Job drawing, mm, ordinate dimensions from the low corner. One solid piece. A direction names the side the tool comes from. Round coordinates to 2 decimals unless told otherwise and drop trailing zeros. Loops run counter-clockwise (first coordinate to the right, second up) from the corner with the lowest first, then second, coordinate; pieces in that order, holes last.
1) Drop a flat-ended pin along its axis: P1, Ø8, axis at x = 47.5, y = 28, coming from the +Z side. Give the stop position or say it passes through.
2) Band-saw the part on C-C, the plane y = 28. Write the cut outline in (x, z).
3) Band-saw the part on D-D, the plane x = 66. Write the cut outline in (y, z) (3 decimals).
4) 3-axis set-ups, long thin cutter, end or side, ignore diameter. For the marked faces 1 and 2: which of +Z, -Z, +X, -X, +Y, -Y reach the whole face in a straight line?
5) Mould opens along X. For the marked faces 3, 4, 5 and 6 say: +X half, -X half, draft (parallel to the pull), parting line (faces both ways), or undercut.
6) Probe line 1 (Y direction, x = 66, z = 2.95); line 2 (Y direction, x = 13, z = 1.65); line 3 (Y direction, x = 38, z = 4.5). List the from-to ranges inside material, lowest first.
7) Band-saw the part on B-B, the plane z = 3.4. Write the cut outline in (x, y).
8) Band-saw the part on A-A, the plane x = 27. Write the cut outline in (y, z), then the cut area to 3 significant figures.
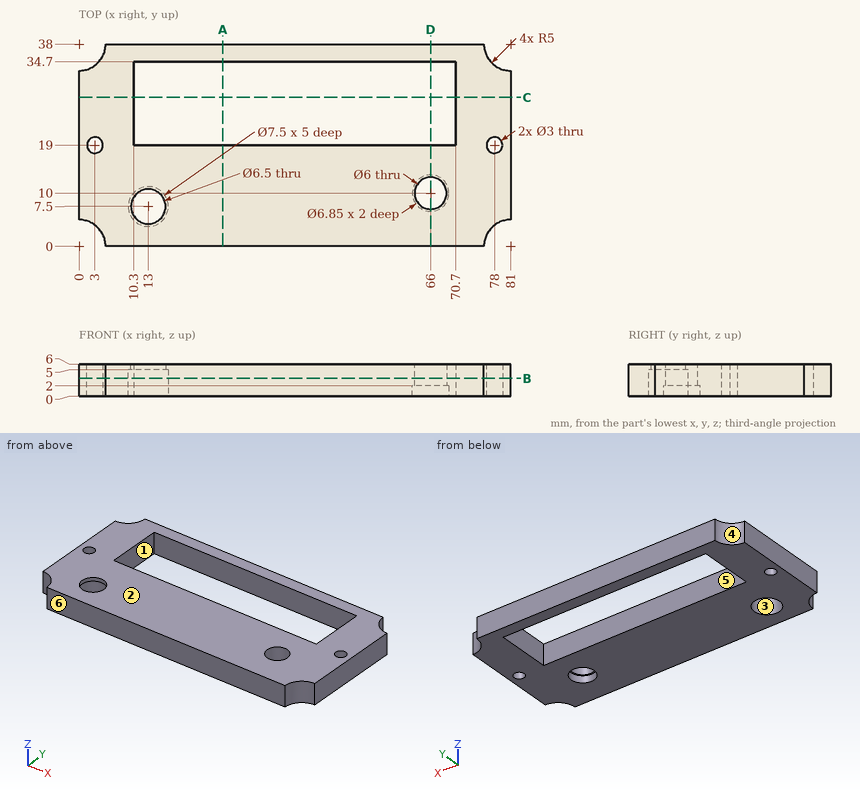
Reported:
1. P1: passes through
2. outline: (0, 0) - (10.3, 0) - (10.3, 6) - (0, 6) - close; (70.7, 0) - (81, 0) - (81, 6) - (70.7, 6) - close
3. outline: (0, 0) - (6.575, 0) - (6.575, 2) - (7, 2) - (7, 6) - (0, 6) - close; (13, 2) - (13.425, 2) - (13.425, 0) - (19, 0) - (19, 6) - (13, 6) - close; (34.7, 0) - (38, 0) - (38, 6) - (34.7, 6) - close
4. face 1: +Z, -Z
4. face 2: +Z, +X, -X, +Y, -Y
5. face 3: undercut
5. face 4: -X half
5. face 5: undercut
5. face 6: draft
6. line 1: y = 0 to 7, 13 to 19, 34.7 to 38
6. line 2: y = 0 to 3.75, 11.25 to 19, 34.7 to 38
6. line 3: y = 0 to 19, 34.7 to 38
7. outline: (0, 5) arc R5 cw to (5, 0) - (76, 0) arc R5 cw to (81, 5) - (81, 33) arc R5 cw to (76, 38) - (5, 38) arc R5 cw to (0, 33) - close; hole circle Ø3 at (3, 19); hole circle Ø7.5 at (13, 7.5); hole (10.3, 19) - (70.7, 19) - (70.7, 34.7) - (10.3, 34.7) - close; hole circle Ø6 at (66, 10); hole circle Ø3 at (78, 19)
8. outline: (0, 0) - (19, 0) - (19, 6) - (0, 6) - close; (34.7, 0) - (38, 0) - (38, 6) - (34.7, 6) - close
8. area: 134 mm2
